from build123d import *

# Parameters (mm, degrees)
F0_R     = 76.51913
F1_DEPTH = 25.4
F2_R     = 7.9375
F3_DEPTH = 50.8
F4_R     = 12.7
F5_DEPTH = 25.4


with BuildPart() as f1:
    # F0 (on Top) → F1 (new body)
    with BuildSketch(Plane.XY):
        Circle(F0_R)
    extrude(amount=F1_DEPTH)

    # F2 (on Top) → F3 (join)
    with BuildSketch(Plane.XY):
        with Locations((-35.814576, 32.962088)):
            Circle(F2_R)
    extrude(amount=F3_DEPTH)

    # F4 (on Top) → F5 (join)
    with BuildSketch(Plane.XY):
        Circle(F4_R)
    extrude(amount=-F5_DEPTH)


solid = f1.part
Geometry check sheet. Reference: the model listing, model coordinates, mm. A direction names the side the tool comes from. Give positions to 0.01 mm unless a question says otherwise; leave off trailing zeros. Order: outer loops, then holes, each group sorted by start corner. A loop starts at its lowest first (then second) coordinate and runs counter-clockwise, first axis right, second up. Notation, with made-up numbers: (77, 56.25) - (87, 56.25) arc R33 cw to (87, 84.25) - close; hole circle Ø8 at (9.25, 44.25). An arc over 180 degrees is marked (long way). Use one line per item in the form item = value.
1) Sectioned sample at A-A (x = 0). Record the boundary of the cut face in (y, z).
Working result:
outline = (-76.52, 0) - (-12.7, 0) - (-12.7, -25.4) - (12.7, -25.4) - (12.7, 0) - (76.52, 0) - (76.52, 25.4) - (-76.52, 25.4) - close
2) Sectioned sample at D-D (y = 50.5). Record the boundary of the cut face in (x, z).
Working result:
outline = (-57.49, 0) - (57.49, 0) - (57.49, 25.4) - (-57.49, 25.4) - close
3) Material ranges on probe 1 along Z at (x, y) = (45, 45.5); probe 2 along Y at (x, z) = (65, 18); probe 3 along X at (y, z) = (4.5, 19), recorded low to high. Write a range as from..to.
Working result:
probe_1 = 0..25.4
probe_2 = -40.38..40.38
probe_3 = -76.39..76.39
4) Access from +Z, -Z, +X, -X, +Y, -Y to the whole of each face (thin tool, end or side, straight path). Record for faces 1 (the face through (-41.66, 38.33, 37.92)), 2 (the face through (-2.75, -12.4, -12.52)), 3 (the face through (-60.723, -46.561, 12.522)).
Working result:
face_1 = +Z
face_2 = -Z
face_3 = +Z, -Z
5) Sectioned sample at C-C (z = 23). Record the boundary of the cut face in (x, y), and give its area (3 significant figures).
Working result:
outline = circle Ø153.04 at (0, 0)
area = 18,400 mm^2
6) Depth check by flat-ended pin: pin 1 Ø12 at (y, z) = (-36.5, 24.5) entering from -X; pin 2 Ø10 at (y, z) = (59.5, 11.5) entering from +X; pin 3 Ø6 at (x, y) = (-37.5, -40.5) entering from +Z; pin 4 Ø8 at (y, z) = (54, 30) entering from -X. Enter the tip coordinate at first touch or a pass-through.
Working result:
pin_1 = -70.18
pin_2 = 53.71
pin_3 = 25.4
pin_4 = through
